from build123d import *

# Parameters (mm, degrees)
F1_DEPTH = 25.4


with BuildPart() as f1:
    # F0 (on Front) → F1 (new body)
    with BuildSketch(Plane.XZ):
        Polygon((-88.257447, -59.687648), (-82.12845, -49.147233), (-134.837762, -49.147233), (-143.809088, -14.351459), (-125.996976, -4.606415), (-88.257447, 16.040962), (-76.612361, 30.896192), (-149.547338, 0), (-149.547338, -59.687648), align=None)
        Polygon((-134.837762, -49.147233), (-82.12845, -49.147233), (-9.55318, -49.147233), (-9.55318, 16.040962), (-88.257447, 16.040962), (-94.386436, -31.234344), (-125.996976, -4.606415), (-143.809088, -14.351459), align=None)
        Polygon((-88.257447, 16.040962), (-9.55318, 16.040962), (17.77407, 52.627109), (-29.419146, 45.1326), (-76.612361, 30.896192), align=None)
    extrude(amount=F1_DEPTH)


solid = f1.part
Part model, mm, in its own coordinate system. A direction names the side the tool comes from. Coordinates: 2 decimals unless noted, no trailing zeros. Loops run counter-clockwise (first coordinate to the right, second up) from the corner with the lowest first, then second, coordinate; pieces in that order, holes last. Notation, with made-up numbers: M 46,20 L 93,20 A11 ccw 93,31 Z; hole C -24.75,88.5 d5. An arc over 180 degrees is marked long. Use a Markdown table: item, result. Add a question column.
Q1. Mould opens along Z. For faces 4 (the flat face through (-107.391, -12.522, 5.573)), 5 (the flat face through (3.92, -12.52, 34.08)), 6 (the flat face through (-5.492, -12.522, 48.932)) say: +Z half, -Z half, draft (parallel to the pull), parting line (faces both ways), or undercut.
Q2. Pin check, flat tips, straight feed: P1, Ø12, axis at x = -9, z = 37.5, coming from the +Y side; P2, Ø1, axis at x = -74, y = -13, coming from the +Z side; P3, Ø12.5, axis at y = -6.5, z = -15.5, coming from the +X side; P4, Ø8, axis at x = -94.5, y = -12.5, coming from the +Z side. Stop position of each tip, or through.
Q3. Which spindle directions (+Z, -Z, +X, -X, +Y, -Y) get a long thin tool onto all of the face, cutting with end or side? Do faces 1 (the flat face through (-52.685, -12.522, 38.114)), 2 (the flat face through (-9.553, -13, -17)), 3 (the flat face through (-91.28, -12.52, -7.27)). Say none if no direction does.
Q4. Cut at B-B (z = -11.5). Write the cut outline in (x, y).
Q5. Cut at C-C (y = -18). Write the cut outline in (x, z).
Q6. Cut at D-D (z = -47). Write the cut outline in (x, y).
Q7. Cut at A-A (x = -124). Write the cut outline in (y, z), and give its area (3 significant figures).
Q8. Probe L1, parallel to X at y = -10.75, z = -39.5; L2, parallel to Z at x = -104, y = -2.5; L3, parallel to X at y = -17.5, z = -14.5. List the from-to ranges inside material, lowest first.
Worked out:
| question | item | result |
|---|---|---|
| 1 | face 4 | undercut |
| 1 | face 5 | -Z half |
| 1 | face 6 | +Z half |
| 2 | P1 | stops at y = 0 |
| 2 | P2 | stops at z = 31.84 |
| 2 | P3 | stops at x = -9.55 |
| 2 | P4 | stops at z = 25.01 |
| 3 | face 1 | +Z, -X, +Y, -Y |
| 3 | face 2 | -Z, +X, +Y, -Y |
| 3 | face 3 | +Y, -Y |
| 4 | outline | M -149.55,-25.4 L -117.81,-25.4 L -117.81,0 L -149.55,0 Z; M -91.83,-25.4 L -9.55,-25.4 L -9.55,0 L -91.83,0 Z |
| 5 | outline | M -149.55,-59.69 L -88.26,-59.69 L -82.13,-49.15 L -9.55,-49.15 L -9.55,16.04 L 17.77,52.63 L -29.42,45.13 L -76.61,30.9 L -149.55,0 Z; hole M -126,-4.61 L -94.39,-31.23 L -88.26,16.04 Z |
| 6 | outline | M -149.55,-25.4 L -9.55,-25.4 L -9.55,0 L -149.55,0 Z |
| 7 | outline | M -25.4,-59.69 L 0,-59.69 L 0,-6.29 L -25.4,-6.29 Z; M -25.4,-3.51 L 0,-3.51 L 0,10.82 L -25.4,10.82 Z |
| 7 | area | 1,720 mm2 |
| 8 | L1 | x = -149.55 to -9.55 |
| 8 | L2 | z = -59.69 to -23.14, 7.43 to 19.29 |
| 8 | L3 | x = -149.55 to -114.25, -92.22 to -9.55 |
